CAD build for the part. Positions are in the model's coordinates, mm. A direction names the side the tool comes from. Round coordinates to 2 decimals unless told otherwise and drop trailing zeros. Loops run counter-clockwise (first coordinate to the right, second up) from the corner with the lowest first, then second, coordinate; pieces in that order, holes last. Notation, with made-up numbers: (42.5, -9.75) - (63.5, -9.75) arc R17 ccw to (63.5, -2.75) - close; hole circle Ø1 at (-39.5, 21). An arc over 180 degrees is marked (long way). One line per question, with ' | ' between items.
Autodesk Fusion 360 part; units mm, degrees
sketch "Sketch1" plane through (0, 0, 0) normal (1, 0, 0) x (0, 1, 0)
  circle A0 centre (0, 0) radius 29.075
  circle A1 centre (0, 0) radius 31.75
  dimension "d1" = 58.15
  dimension "d2" = 63.5
extrude "Extrude1" add sketch "Sketch1" along normal blind 38.1
ref_plane "WorkPlane1" through (76.2, 0, 0) normal (1, 0, 0) x (0, 1, 0)
sketch "Sketch2" plane through (76.2, 0, 0) normal (1, 0, 0) x (0, 1, 0)
  line L0 (-63.5, -31.75) -> (63.5, -31.75)
  line L1 (63.5, -31.75) -> (63.5, 12.7)
  line L2 (63.5, 12.7) -> (-63.5, 12.7)
  line L3 (-63.5, 12.7) -> (-63.5, -31.75)
  circle A0 centre (0, 0) radius 31.75 construction
  line L4 (-60.325, -26.67) -> (60.325, -26.67)
  line L5 (60.325, -26.67) -> (60.325, 9.525)
  line L6 (60.325, 9.525) -> (-60.325, 9.525)
  line L7 (-60.325, 9.525) -> (-60.325, -26.67)
  dimension "d6" = 63.5
  dimension "d7" = 63.5
  dimension "d8" = 44.45
sketch "Sketch3" plane through (38.1, 0, 0) normal (1, 0, 0) x (0, 1, 0)
  line L0 (0, 0) -> (-24.2467, -24.2467) construction
  arc A0 (-20.2056, 20.2056) -> (-20.2056, -20.2056) centre (0, 0) ccw
  arc A1 (20.2056, 20.2056) -> (-20.2056, 20.2056) centre (0, 0) ccw
  arc A2 (20.2056, -20.2056) -> (20.2056, 20.2056) centre (0, 0) ccw
  arc A3 (-20.2056, -20.2056) -> (20.2056, -20.2056) centre (0, 0) ccw
  arc A4 (-22.4506, 22.4506) -> (-22.4506, -22.4506) centre (0, 0) ccw
  line L1 (0, 0) -> (-22.4506, 22.4506) construction
  line L2 (0, 0) -> (-22.4506, -22.4506) construction
  arc A5 (22.4506, 22.4506) -> (-22.4506, 22.4506) centre (0, 0) ccw
  line L3 (0, 0) -> (22.4506, 22.4506) construction
  line L4 (0, 0) -> (-22.4506, 22.4506) construction
  arc A6 (22.4506, -22.4506) -> (22.4506, 22.4506) centre (0, 0) ccw
  line L5 (0, 0) -> (22.4506, -22.4506) construction
  line L6 (0, 0) -> (22.4506, 22.4506) construction
  arc A7 (-22.4506, -22.4506) -> (22.4506, -22.4506) centre (0, 0) ccw
  dimension "d10" = 28.575
  dimension "d11" = 31.75
  dimension "d12" = 90
  dimension "d13" = 90
  dimension "d14" = 90
loft "Loft1" add profiles "Sketch3", "Sketch2" section 1 section 2
loft "Loft2" cut profiles "Sketch3", "Sketch2" section 1 contours A0 A1 A2 A3 section 2 contours L4 L5 L6 L7
extrude "Extrude2" add sketch "Sketch2" along normal blind 25.4
sketch "Sketch4" plane through (0, 0, -26.67) normal (0, 0, -1) x (1, 0, 0)
  circle A0 centre (86.36, 38.1) radius 9.65
  circle A1 centre (86.36, -38.1) radius 9.65
  line L0 (76.2, 63.5) -> (101.6, 63.5) construction
  line L1 (76.2, -63.5) -> (101.6, -63.5) construction
  line L2 (86.36, 63.5) -> (86.36, -63.5) construction
  circle A2 centre (86.36, 12.7) radius 9.65
  circle A3 centre (86.36, -12.7) radius 9.65
  dimension "d18" = 19.3
  dimension "d20" = 19.3
  dimension "d28" = 19.3
  dimension "d29" = 19.3
  dimension "d30" = 25.4
  dimension "d31" = 25.4
  dimension "d32" = 25.4
  dimension "d33" = 25.4
  dimension "d35" = 10.16
extrude "Extrude3" cut sketch "Sketch4" along normal blind 4.175
chamfer "Chamfer1" distance 5.08 distance2 3.81 1 edges at (101.6, 0, -26.67) measured on face at (101.6, 20.1083, -30.0567)
equation "d1 = 2.25 in + 1 mm"
equation "d2 = 2.25 in + 0.25 in"
equation "d18 = magnetDiameter + magnetClearance"
equation "d20 = magnetDiameter + magnetClearance"
equation "d25 = magnetHeight + 1 mm"
equation "d28 = magnetDiameter + magnetClearance"
equation "d29 = magnetDiameter + magnetClearance"
equation "magnetDiameter = 0.75 in"
equation "magnetClearance = 0.25 mm"
equation "magnetHeight = ( 1 / 8 ) * 1 in"
(1) Cut at B-B, the plane x = 24.5. Write the cut outline in (y, z) (3 decimals).
Results found:
outline: circle Ø63.5 at (0, 0); hole circle Ø58.15 at (0, 0)
(2) Two-plate mould, pull along Z, no slides. Class faces 4 (the face through (86, -13, -30.845)), 5 (the face through (89, 63.5, -10)), 6 (the face through (18.783, -6.883, 30.995)): released by +Z, released by -Z, zero draft, split by the parting line, or undercut.
Results found:
face 4: undercut | face 5: zero draft | face 6: split by the parting line
(3) Probe L1, parallel to Y at x = 86.36, z = -29.7; L2, parallel to Z at x = 85.5, y = -23 (3 decimals); L3, parallel to Y at x = 89, z = 8 (3 decimals). List the from-to ranges inside material, lowest first.
Results found:
L1: y = -63.5 to -47.75, -28.45 to -22.35, -3.05 to 3.05, 22.35 to 28.45, 47.75 to 63.5 | L2: z = -31.75 to -26.67, 9.525 to 12.7 | L3: y = -63.5 to -60.325, 60.325 to 63.5
(4) Tool access for faces 1 (the face through (89, 60.325, -7)), 2 (the face through (38.1, 28.74, 1.52)), 3 (the face through (79.248, -6.178, -28.728)): list every direction of +Z, -Z, +X, -X, +Y, -Y with a clear straight run to the whole face (end or side of a thin tool).
Results found:
face 1: +X | face 2: -X | face 3: none
(5) Drop flat-ended pins along their axis: P1, Ø1.5, axis at x = 67.5, y = 10, coming from the +Z side; P2, Ø11.5, axis at x = 86.36, y = -38.1, coming from the +Z side; P3, Ø8, axis at x = 25, y = 31.5, coming from the +Z side. Give the stop position or say it passes through.
Results found:
P1: stops at z = 17.34 | P2: stops at z = 12.7 | P3: stops at z = 15.87
(6) Cut at A-A, the plane x = 86.36. Write the cut outline in (y, z) (3 decimals).
Results found:
outline: (-63.5, -31.75) - (63.5, -31.75) - (63.5, 12.7) - (-63.5, 12.7) - close; hole (-60.325, -26.67) - (-47.75, -26.67) - (-47.75, -30.845) - (-28.45, -30.845) - (-28.45, -26.67) - (-22.35, -26.67) - (-22.35, -30.845) - (-3.05, -30.845) - (-3.05, -26.67) - (3.05, -26.67) - (3.05, -30.845) - (22.35, -30.845) - (22.35, -26.67) - (28.45, -26.67) - (28.45, -30.845) - (47.75, -30.845) - (47.75, -26.67) - (60.325, -26.67) - (60.325, 9.525) - (-60.325, 9.525) - close
